from build123d import *

# Parameters (mm, degrees)
BOSS_EXTRUDE1_DEPTH                              = 7
CBORE_FOR_M3_PAN_HEAD_MACHINE_SCREW1_D           = 3.2
CBORE_FOR_M3_PAN_HEAD_MACHINE_SCREW1_CBORE_D     = 7
CBORE_FOR_M3_PAN_HEAD_MACHINE_SCREW1_CBORE_DEPTH = 2.4
SKETCH5_R                                        = 9.5
CUT_EXTRUDE1_DEPTH                               = 1
CUT_EXTRUDE1_DEPTH_BACK                          = 8
SKETCH6_R                                        = 3.5
CUT_EXTRUDE2_DEPTH                               = 1
CUT_EXTRUDE2_DEPTH_BACK                          = 8
SKETCH7_R                                        = 9.5
CUT_EXTRUDE3_DEPTH                               = 1
CUT_EXTRUDE3_DEPTH_BACK                          = 8


with BuildPart() as part:
    # Sketch1 → Boss-Extrude1 (new body)
    with BuildSketch(Plane(origin=(0, 0, 0), x_dir=(0, 0, -1), z_dir=(1, 0, 0))):
        with BuildLine():
            ThreePointArc((77.801960973, 11), (73, 0), (77.801960973, -11))
            Line((77.801960973, -11), (88, -11))
            Line((88, -11), (88, 11))
            Line((88, 11), (77.801960973, 11))
        make_face()
        with BuildLine():
            Line((88, -11), (77.801960973, -11))
            ThreePointArc((77.801960973, -11), (94.001225483, -13.747192175), (103, 0))
            ThreePointArc((103, 0), (94.001225483, 13.747192175), (77.801960973, 11))
            Line((77.801960973, 11), (88, 11))
            Line((88, 11), (88, -11))
        make_face()
        with BuildLine():
            ThreePointArc((22, 0), (21.250368178, -5.694018992), (19.052558883, -11))
            Line((19.052558883, -11), (77.801960973, -11))
            ThreePointArc((77.801960973, -11), (73, 0), (77.801960973, 11))
            Line((77.801960973, 11), (19.052558883, 11))
            ThreePointArc((19.052558883, 11), (21.250368178, 5.694018992), (22, 0))
        make_face()
        with BuildLine():
            Line((0, 11), (0, -11))
            Line((0, -11), (19.052558883, -11))
            ThreePointArc((19.052558883, -11), (21.250368178, -5.694018992), (22, 0))
            ThreePointArc((22, 0), (21.250368178, 5.694018992), (19.052558883, 11))
            Line((19.052558883, 11), (0, 11))
        make_face()
        with BuildLine():
            Line((19.052558883, -11), (0, -11))
            Line((0, -11), (0, 11))
            Line((0, 11), (19.052558883, 11))
            ThreePointArc((19.052558883, 11), (-22, 0), (19.052558883, -11))
        make_face()
    extrude(amount=BOSS_EXTRUDE1_DEPTH)

    # CBORE for M3 Pan Head Machine Screw1 (through all)
    with Locations(Plane(origin=(7, 0, 0), x_dir=(0, 0, -1), z_dir=(1, 0, 0))):
        with Locations((0, -17.5), (0, 17.5), (-17.5, 0)):
            CounterBoreHole(CBORE_FOR_M3_PAN_HEAD_MACHINE_SCREW1_D / 2, CBORE_FOR_M3_PAN_HEAD_MACHINE_SCREW1_CBORE_D / 2, CBORE_FOR_M3_PAN_HEAD_MACHINE_SCREW1_CBORE_DEPTH)

    # Sketch5 → Cut-Extrude1 (cut, two sides)
    with BuildSketch(Plane(origin=(7, 0, 0), x_dir=(0, 0, -1), z_dir=(1, 0, 0))) as cut_extrude1_sk:
        Circle(SKETCH5_R)
    extrude(amount=CUT_EXTRUDE1_DEPTH, mode=Mode.SUBTRACT)
    extrude(cut_extrude1_sk.sketch, amount=-CUT_EXTRUDE1_DEPTH_BACK, mode=Mode.SUBTRACT)

    # Sketch6 → Cut-Extrude2 (cut, two sides)
    with BuildSketch(Plane(origin=(7, 0, 0), x_dir=(0, 0, -1), z_dir=(1, 0, 0))) as cut_extrude2_sk:
        with Locations((15.556349186, 15.556349186)):
            Circle(SKETCH6_R)
        with Locations((-15.556349186, 15.556349186)):
            Circle(SKETCH6_R)
        with Locations((-15.556349186, -15.556349186)):
            Circle(SKETCH6_R)
        with Locations((15.556349186, -15.556349186)):
            Circle(SKETCH6_R)
    extrude(amount=CUT_EXTRUDE2_DEPTH, mode=Mode.SUBTRACT)
    extrude(cut_extrude2_sk.sketch, amount=-CUT_EXTRUDE2_DEPTH_BACK, mode=Mode.SUBTRACT)

    # Sketch7 → Cut-Extrude3 (cut, two sides)
    with BuildSketch(Plane(origin=(7, 0, 0), x_dir=(0, 0, -1), z_dir=(1, 0, 0))) as cut_extrude3_sk:
        with Locations((88, 0)):
            Circle(SKETCH7_R)
    extrude(amount=CUT_EXTRUDE3_DEPTH, mode=Mode.SUBTRACT)
    extrude(cut_extrude3_sk.sketch, amount=-CUT_EXTRUDE3_DEPTH_BACK, mode=Mode.SUBTRACT)


solid = part.part
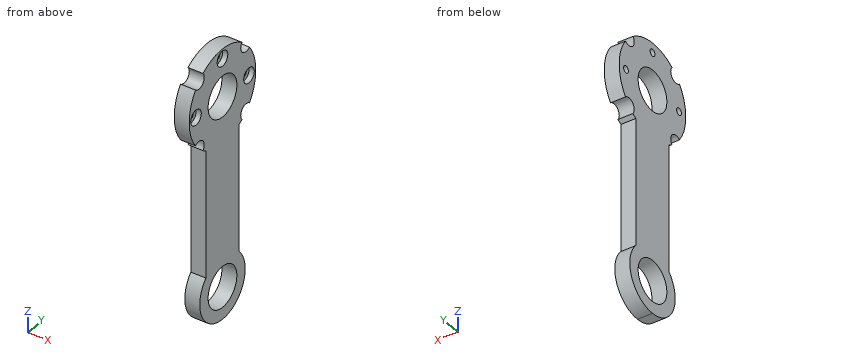
Verification items for the finished model (mm, model axes). Coordinates: 2 decimals unless noted, no trailing zeros. Write each loop counter-clockwise with the first axis right and the second up, starting at its lowest first coordinate (ties: lowest second). Pieces come first, ordered by that corner, then holes. Notation, with made-up numbers: M 68.5,-18.75 L 122.5,-18.75 A15 cw 122.5,-8.75 Z; hole C 81.25,-36 d7. An arc over 180 degrees is marked long. Use a Markdown table: item, result.
Q1. Go/stop test with flat-tipped pins: P1, Ø4, axis at y = -5.5, z = -78.5, coming from the -X side; P2, Ø3.5, axis at y = 0, z = 17.5, coming from the +X side; P3, Ø2, axis at x = 5.5, z = -57, coming from the +Y side; P4, Ø4, axis at x = 5.5, y = 15.5, coming from the -Z side. Record where each tip stops, or that it passes through.
Reply:
| item | result |
|---|---|
| P1 | stops at x = 0 |
| P2 | stops at x = 4.6 |
| P3 | stops at y = 11 |
| P4 | stops at z = -94.54 |
Q2. Sectioned sample at D-D, the plane z = 8. Record the boundary of the cut face in (x, y), plus the area to 3 significant figures.
Reply:
| item | result |
|---|---|
| outline | M 0,-20.49 L 7,-20.49 L 7,-5.12 L 0,-5.12 Z; M 0,5.12 L 7,5.12 L 7,20.49 L 0,20.49 Z |
| area | 215 mm² |
Q3. Thickness scan on line 1 (Z direction, x = 3.25, y = -3); line 2 (Z direction, x = 3.5, y = -12); line 3 (Y direction, x = 2, z = -63.5). Record the ranges inside material, lowest first.
Reply:
| item | result |
|---|---|
| line 1 | z = -102.7 to -97.01, -78.99 to -9.01, 9.01 to 21.79 |
| line 2 | z = -97 to -79, -18.44 to 18.44 |
| line 3 | y = -11 to 11 |
Q4. Sectioned sample at A-A, the plane z = -88. Record the boundary of the cut face in (x, y).
Reply:
| item | result |
|---|---|
| outline | M 0,-15 L 7,-15 L 7,-9.5 L 0,-9.5 Z; M 0,9.5 L 7,9.5 L 7,15 L 0,15 Z |
Q5. Sectioned sample at C-C, the plane y = -7.5. Record the boundary of the cut face in (x, z), plus the area to 3 significant figures.
Reply:
| item | result |
|---|---|
| outline | M 0,-100.99 L 7,-100.99 L 7,-93.83 L 0,-93.83 Z; M 0,-82.17 L 7,-82.17 L 7,-5.83 L 0,-5.83 Z; M 0,5.83 L 7,5.83 L 7,20.68 L 0,20.68 Z |
| area | 688 mm² |
Q6. Sectioned sample at B-B, the plane x = 3.5. Record the boundary of the cut face in (y, z), plus the area to 3 significant figures.
Reply:
| item | result |
|---|---|
| outline | M -17.83,-12.89 A3.5 cw -12.89,-17.83 A22 ccw -11,-19.05 L -11,-77.8 A15 ccw long 11,-77.8 L 11,-19.05 A22 ccw 12.89,-17.83 A3.5 cw 17.83,-12.89 A22 ccw 17.83,12.89 A3.5 cw 12.89,17.83 A22 ccw -12.89,17.83 A3.5 cw -17.83,12.89 A22 ccw Z; hole C -17.5,0 d3.2; hole C 0,-88 d19; hole C 0,0 d19; hole C 0,17.5 d3.2; hole C 17.5,0 d3.2 |
| area | 2,740 mm² |
